Build history of the part. All positions in model axes, mm. A direction names the side the tool comes from. Round coordinates to 2 decimals unless told otherwise and drop trailing zeros. Write each loop counter-clockwise with the first axis right and the second up, starting at its lowest first coordinate (ties: lowest second). Pieces come first, ordered by that corner, then holes.
Item 1: Drop flat-ended pins along their axis: pin 1 Ø3.5 at (x, y) = (27.5, 36.5) entering from -Z; pin 2 Ø0.6 at (x, z) = (-7, -1) entering from +Y; pin 3 Ø0.6 at (y, z) = (3.5, -1) entering from -X; pin 4 Ø1 at (x, z) = (-21.5, -1) entering from +Y. Give the stop position or say it passes through.
Item 2: 3-axis set-ups, long thin cutter, end or side, ignore diameter. For faces 1 (the flat face through (30.5, -1, 1)), 2 (the flat face through (0, -39.5, 1)), 3 (the flat face through (-1.8, 3, -1)), 4 (the flat face through (-14.5, 3, 0)), 5 (the flat face through (-10, 10.9, -1)): which of +Z, -Z, +X, -X, +Y, -Y reach the whole face in a straight line?
Item 3: Band-saw the part on D-D, the plane y = 2.95. Write the cut outline in (x, z), then the cut area to 3 significant figures.
Item 4: Wall check: probe 1 along Y at (x, z) = (27.5, 2); probe 2 along Y at (x, z) = (-6, -1.3); probe 3 along Y at (x, z) = (-8, 1.75). Give the ranges that are in metal, low to high.
Item 5: Band-saw the part on B-B, the plane x = 27.5. Write the cut outline in (y, z), then the cut area to 3 significant figures.
Item 6: Mould opens along X. For faces 6 (the flat face through (-17, 3, -1)), 7 (the cylindrical face through (-26.831, 35.214, 1.479)), 8 (the flat face through (-9, -2.5, 0)), 9 (the flat face through (0, 1, 0)) say: +X half, -X half, draft (parallel to the pull), parting line (faces both ways), or undercut.
Item 7: Band-saw the part on C-C, the plane x = -7. Write the cut outline in (y, z), then the cut area to 3 significant figures.
Item 8: Band-saw the part on A-A, the plane y = -36.5. Write the cut outline in (x, z).
```python
from build123d import *

# Parameters (mm, degrees)
F0_W     = 61
F0_H     = 79
F0_R     = 1.45
F0_W_2   = 15.200002
F0_H_2   = 15.900002
F0_W_3   = 10.2
F0_H_3   = 10.9
F0_R_2   = 3.3
F1_DEPTH = 3
F2_DEPTH = 1.9
F3_DEPTH = 1.9


with BuildPart() as f1:
    # F0 (on Top) → F1 (new body)
    with BuildSketch(Plane.XY):
        Rectangle(F0_W, F0_H)
        with Locations((-27.5, -36.5)):
            Circle(F0_R, mode=Mode.SUBTRACT)
        with Locations((27.5, -36.5)):
            Circle(F0_R, mode=Mode.SUBTRACT)
        with Locations((-9.4, 2.95)):
            Rectangle(F0_W_2, F0_H_2, mode=Mode.SUBTRACT)
        with Locations((-27.5, 36.5)):
            Circle(F0_R, mode=Mode.SUBTRACT)
        with Locations((27.5, 36.5)):
            Circle(F0_R, mode=Mode.SUBTRACT)
        with Locations((-9.4, 2.95)):
            Rectangle(F0_W_2, F0_H_2)
        with Locations((-9.4, 2.95)):
            Rectangle(F0_W_3, F0_H_3, mode=Mode.SUBTRACT)
        with Locations((-9.4, 2.95)):
            Rectangle(F0_W_3, F0_H_3)
        with Locations((-9.4, 2.95)):
            Circle(F0_R_2, mode=Mode.SUBTRACT)
    extrude(amount=F1_DEPTH)

    # F0 (on Top) → F2 (cut)
    with BuildSketch(Plane.XY):
        with Locations((-9.4, 2.95)):
            Rectangle(F0_W_3, F0_H_3)
        with Locations((-9.4, 2.95)):
            Circle(F0_R_2, mode=Mode.SUBTRACT)
    extrude(amount=F2_DEPTH, mode=Mode.SUBTRACT)

    # F0 (on Top) → F3 (join)
    with BuildSketch(Plane.XY):
        with Locations((-9.4, 2.95)):
            Rectangle(F0_W_2, F0_H_2)
        with Locations((-9.4, 2.95)):
            Rectangle(F0_W_3, F0_H_3, mode=Mode.SUBTRACT)
    extrude(amount=-F3_DEPTH)


solid = f1.part
```
Results:
1. pin 1: stops at z = 0
1. pin 2: stops at y = 10.9
1. pin 3: stops at x = -17
1. pin 4: passes through
2. face 1: +Z, -Z, +X, +Y, -Y
2. face 2: +Z, -Z, +X, -X, -Y
2. face 3: -Z, +X, +Y, -Y
2. face 4: -Z
2. face 5: -Z, +X, -X, +Y
3. outline: (-30.5, 0) - (-17, 0) - (-17, -1.9) - (-14.5, -1.9) - (-14.5, 1.9) - (-12.7, 1.9) - (-12.7, 3) - (-30.5, 3) - close; (-6.1, 1.9) - (-4.3, 1.9) - (-4.3, -1.9) - (-1.8, -1.9) - (-1.8, 0) - (30.5, 0) - (30.5, 3) - (-6.1, 3) - close
3. area: 166 mm2
4. probe 1: y = -39.5 to -37.95, -35.05 to 35.05, 37.95 to 39.5
4. probe 2: y = -5 to -2.5, 8.4 to 10.9
4. probe 3: y = -39.5 to -2.5, 8.4 to 39.5
5. outline: (-39.5, 0) - (-37.95, 0) - (-37.95, 3) - (-39.5, 3) - close; (-35.05, 0) - (35.05, 0) - (35.05, 3) - (-35.05, 3) - close; (37.95, 0) - (39.5, 0) - (39.5, 3) - (37.95, 3) - close
5. area: 220 mm2
6. face 6: -X half
6. face 7: undercut
6. face 8: undercut
6. face 9: draft
7. outline: (-39.5, 0) - (-5, 0) - (-5, -1.9) - (-2.5, -1.9) - (-2.5, 1.9) - (0.69, 1.9) - (0.69, 3) - (-39.5, 3) - close; (5.21, 1.9) - (8.4, 1.9) - (8.4, -1.9) - (10.9, -1.9) - (10.9, 0) - (39.5, 0) - (39.5, 3) - (5.21, 3) - close
7. area: 221 mm2
8. outline: (-30.5, 0) - (-28.95, 0) - (-28.95, 3) - (-30.5, 3) - close; (-26.05, 0) - (26.05, 0) - (26.05, 3) - (-26.05, 3) - close; (28.95, 0) - (30.5, 0) - (30.5, 3) - (28.95, 3) - close
